Model file for the job. Use its own axes, mm. A direction names the side the tool comes from. Round coordinates to 2 decimals unless told otherwise and drop trailing zeros. Order: outer loops, then holes, each group sorted by start corner. A loop starts at its lowest first (then second) coordinate and runs counter-clockwise, first axis right, second up. Notation, with made-up numbers: (21.5, 79.25) -> (56.5, 79.25) arc R19 ccw to (56.5, 90.25) -> close; hole circle Ø8 at (32.5, 57.25). An arc over 180 degrees is marked (long way). Put each result on its own line as item: value. Start each with the question number.
Q1. 3-axis set-ups, long thin cutter, end or side, ignore diameter. For faces 1 (the face through (-42.127, -6.926, 13.983)), 2 (the face through (-39.592, -7, 8)), 3 (the face through (-44.592, -7, 8)): which of +Z, -Z, +X, -X, +Y, -Y reach the whole face in a straight line?
Q2. Cut at C-C, the plane x = -33.25. List the corners of the cut face in (y, z), and give its area (3 significant figures).
Q3. Cut at B-B, the plane z = 10.5. List the corners of the cut face in (x, y).
Q4. Cut at D-D, the plane y = -9.5. List the corners of the cut face in (x, z), and give its area (3 significant figures).
Q5. Flat gauge pin, fed straight in: P1, Ø5, axis at x = -47.5, y = -5.5, coming from the +Z side. Where does the tip first touch, or does it go through?
Q6. Probe L1, parallel to Z at x = -52.75, y = -11.25; L2, parallel to X at y = -10.25, z = 5.5; L3, parallel to Z at x = -40.25, y = -6. List the from-to ranges inside material, lowest first.
Q7. Pull direction Y, two halves, no side cores. Call faces 4 (the face through (-51.59, -7.1, 1.52)), 5 (the face through (-42.057, -3.612, 15.496)), 6 (the face through (-37, -7, 3)): released by +Y, released by -Y, zero draft, split by the parting line, or undercut.
from build123d import *

# Parameters (mm, degrees)
F0_W     = 25
F0_H     = 10
F1_DEPTH = 3
F2_W     = 5
F2_H     = 10
F3_DEPTH = 14
F5_R     = 4.99999
F4_R     = 2
F7_DEPTH = 3
F6_R     = 2
F8_DEPTH = 5


# Not quite as in the source:
# - a fillet or chamfer is up to 0.001 mm smaller than in the source, because OpenCascade refuses the exact size


with BuildPart() as f1:
    # F0 (on Top) → F1 (new body)
    with BuildSketch(Plane.XY):
        with Locations((-42.0921362936, -7.1861277148)):
            Rectangle(F0_W, F0_H)
    extrude(amount=F1_DEPTH)

    # F2 (on face) → F3 (join)
    with BuildSketch(Plane.XY.offset(3)):
        with Locations((-42.0921362936, -7.1861277148)):
            Rectangle(F2_W, F2_H)
    extrude(amount=F3_DEPTH)

    # F5 (radius 5 in the source; OpenCascade refuses exactly that, so slightly less here)
    f5_edges = [f1.edges().sort_by_distance(p)[0] for p in [
        (-42.092136, -12.186128, 17),
        (-42.092136, -2.186128, 17),
    ]]
    fillet(f5_edges, radius=F5_R)

    # F4 (on face) → F7 (cut)
    with BuildSketch(Plane.XY.offset(3)):
        with Locations((-49.5921362936, -7.1861277148)):
            Circle(F4_R)
        with Locations((-34.5921362936, -7.1861277148)):
            Circle(F4_R)
    extrude(amount=-F7_DEPTH, mode=Mode.SUBTRACT)

    # F6 (on face) → F8 (cut)
    with BuildSketch(Plane(origin=(-44.5921362936, 0, 0), x_dir=(0, -1, 0), z_dir=(-1, 0, 0))):
        with Locations((7.1861277148, 12)):
            Circle(F6_R)
    extrude(amount=-F8_DEPTH, mode=Mode.SUBTRACT)


solid = f1.part
Ans:
1. face 1: +X, -X
1. face 2: +Z, +X, +Y, -Y
1. face 3: +Z, -X, +Y, -Y
2. outline: (-12.19, 0) -> (-8.67, 0) -> (-8.67, 3) -> (-12.19, 3) -> close; (-5.7, 0) -> (-2.19, 0) -> (-2.19, 3) -> (-5.7, 3) -> close
2. area: 21.1 mm^2
3. outline: (-44.59, -12.19) -> (-39.59, -12.19) -> (-39.59, -8.51) -> (-44.59, -8.51) -> close; (-44.59, -5.86) -> (-39.59, -5.86) -> (-39.59, -2.19) -> (-44.59, -2.19) -> close
4. outline: (-54.59, 0) -> (-29.59, 0) -> (-29.59, 3) -> (-39.59, 3) -> (-39.59, 16.43) -> (-44.59, 16.43) -> (-44.59, 3) -> (-54.59, 3) -> close
4. area: 142 mm^2
5. P1: stops at z = 3
6. L1: z = 0 to 3
6. L2: x = -44.59 to -39.59
6. L3: z = 0 to 10.39, 13.61 to 16.86
7. face 4: undercut
7. face 5: released by +Y
7. face 6: zero draft
